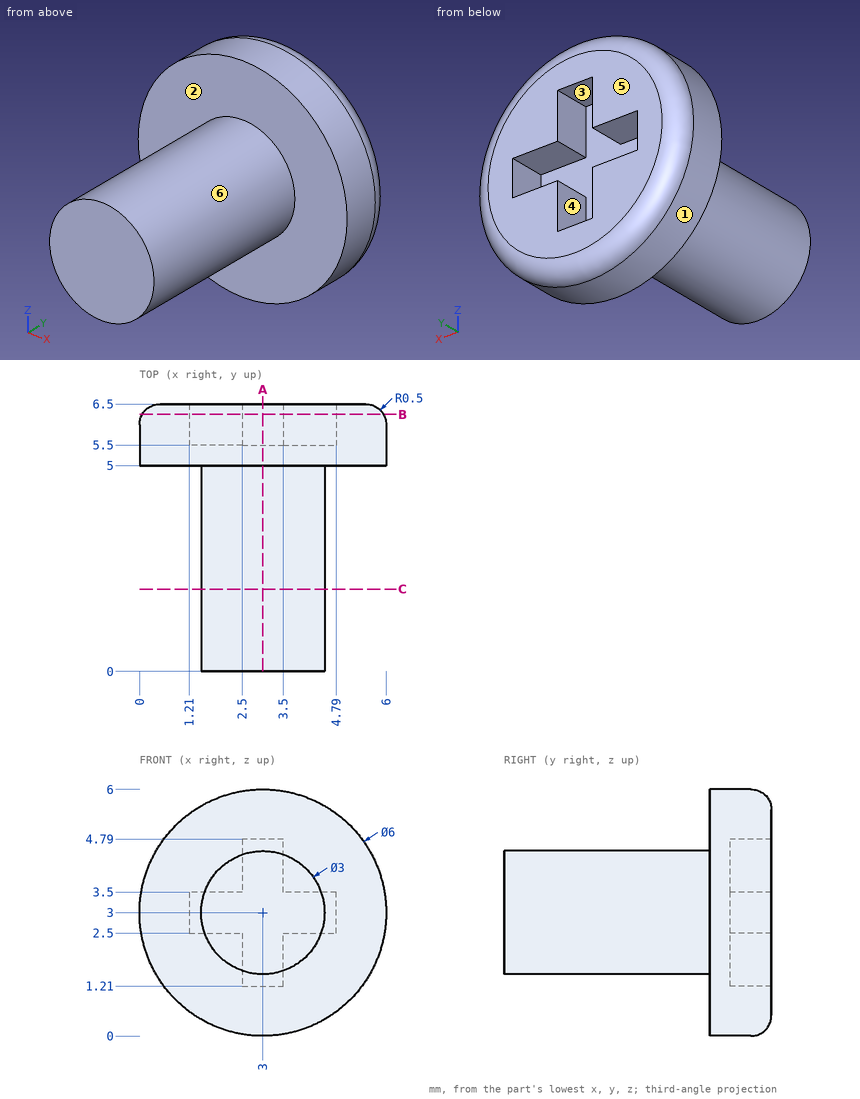
Print and shaded views of the part. All mm, measured from the part's lowest x, y and z. A direction names the side the tool comes from. Round coordinates to 2 decimals unless told otherwise and drop trailing zeros. Loops run counter-clockwise (first coordinate to the right, second up) from the corner with the lowest first, then second, coordinate; pieces in that order, holes last. Notation, with made-up numbers: (14.5, 16.25) -> (68.5, 16.25) arc R25 ccw to (68.5, 31.25) -> close; hole circle Ø7 at (26, 8.25). An arc over 180 degrees is marked (long way). Use CSV: the item, a comma, the result in double quotes. Start each with the question number.
1) Cut at A-A, the plane x = 3. Write the cut outline in (y, z), plus the area to 3 significant figures.
2) Cut at C-C, the plane y = 2. Write the cut outline in (x, z).
3) Wall check: L1, parallel to Y at x = 3, z = 0.5; L2, parallel to Y at x = 2.75, z = 4.75; L3, parallel to X at y = 1.75, z = 3.5 (1 decimal). Give the ranges that are in metal, low to high. Write a range as [from, to].
4) Which spindle directions (+Z, -Z, +X, -X, +Y, -Y) get a long thin tool onto all of the face, cutting with end or side? Do the marked faces 4, 5 and 6. Say none if no direction does.
5) Drop flat-ended pins along their axis: P1, Ø3, axis at x = 2, z = 4, coming from the -Y side; P2, Ø0.5, axis at x = 4, y = 6, coming from the -Z side (1 decimal); P3, Ø0.5, axis at y = 6, z = 2, coming from the -X side (1 decimal); P4, Ø1.1, axis at y = 6, z = 4, coming from the -X side. Give the stop position or say it passes through.
6) Cut at B-B, the plane y = 6.25. Write the cut outline in (x, z).
7) Pull direction Z, two halves, no side cores. Call the marked faces 1, 2 and 3: +Z half, -Z half, draft (parallel to the pull), parting line (faces both ways), or undercut.
Determined:
1,outline,"(0, 1.5) -> (5, 1.5) -> (5, 0) -> (6, 0) arc R0.5 ccw to (6.5, 0.5) -> (6.5, 1.21) -> (5.5, 1.21) -> (5.5, 4.79) -> (6.5, 4.79) -> (6.5, 5.5) arc R0.5 ccw to (6, 6) -> (5, 6) -> (5, 4.5) -> (0, 4.5) -> close"
1,area,"20.3 mm2"
2,outline,"circle Ø3 at (3, 3)"
3,L1,"y = [5, 6.5]"
3,L2,"y = [5, 5.5]"
3,L3,"x = [1.6, 4.4]"
4,face 4,"+Y"
4,face 5,"+Z, -Z, +X, -X, +Y"
4,face 6,"-Y"
5,P1,"stops at y = 0"
5,P2,"stops at z = 0.1"
5,P3,"stops at x = 0.1"
5,P4,"stops at x = 0.03"
6,outline,"circle Ø5.87 at (3, 3); hole (1.21, 2.5) -> (2.5, 2.5) -> (2.5, 1.21) -> (3.5, 1.21) -> (3.5, 2.5) -> (4.79, 2.5) -> (4.79, 3.5) -> (3.5, 3.5) -> (3.5, 4.79) -> (2.5, 4.79) -> (2.5, 3.5) -> (1.21, 3.5) -> close"
7,face 1,"parting line"
7,face 2,"draft"
7,face 3,"undercut"
